Verification items for the finished model (mm, model axes). Give positions to 0.01 mm unless a question says otherwise; leave off trailing zeros. Loops run counter-clockwise (first coordinate to the right, second up) from the corner with the lowest first, then second, coordinate; pieces in that order, holes last. Notation, with made-up numbers: (-24, 49.5) - (10, 49.5) arc R12 cw to (10, 59.5) - close; hole circle Ø8 at (-1.75, 65.5). An arc over 180 degrees is marked (long way). Put each result on its own line as item: value. Start each with the question number.
```python
from build123d import *

# Parameters (mm, degrees)
CHAMFER1_SIZE = 0.5
CHAMFER2_SIZE = 0.5


with BuildPart() as part:
    # Sketch1 → Revolve1 (revolve)
    with BuildSketch(Plane.XY, mode=Mode.PRIVATE) as revolve1_sk:
        with BuildLine():
            Line((5.5, 14.5), (2.236067977, 14.5))
            ThreePointArc((2.236067977, 14.5), (0, 15.5), (-2.236067977, 14.5))
            Line((-2.236067977, 14.5), (-5.5, 14.5))
            Line((-5.5, 14.5), (-5.5, 17.5))
            Line((-5.5, 17.5), (5.5, 17.5))
            Line((5.5, 17.5), (5.5, 14.5))
        make_face()
    revolve(revolve1_sk.sketch.rotate(Axis((-7.5, 0, 0), (1, 0, 0)), 90), axis=Axis((-7.5, 0, 0), (1, 0, 0)))

    # Chamfer1
    chamfer1_edges = [part.edges().sort_by_distance(p)[0] for p in [
        (5.5, 0, -17.5),
        (-5.5, 0, -17.5),
    ]]
    chamfer(chamfer1_edges, length=CHAMFER1_SIZE)

    # Chamfer2
    chamfer2_edges = [part.edges().sort_by_distance(p)[0] for p in [
        (-5.5, 0, -14.5),
        (5.5, 0, -14.5),
    ]]
    chamfer(chamfer2_edges, length=CHAMFER2_SIZE)


solid = part.part
```
1) Section check C-C, the plane x = -2.75. Enter the section's corners in (y, z).
2) Draft check along Y on faces 1 (the face through (0.07, 17.084, -3.794)), 2 (the face through (3.599, 12.864, 6.691)), 3 (the face through (-5.5, 14, -6)). Enter one of: pulls with the +Y half, pulls with the -Y half, needs draft (parallel to the pull), parting line crosses it, or undercut.
3) Scan lines: line 1 along Y through (x, z) = (3.95, 0); line 2 along Y through (x, z) = (3.75, -1.5); line 3 along Z through (x, y) = (2, -6.5). Record each from-to range of solid material in increasing order. Write a range as from..to.
4) Section check A-A, the plane z = 0. Enter the section's corners in (x, y).
5) Depth check by flat-ended pin: P1, Ø5, axis at y = 6.5, z = 10, coming from the -X side; P2, Ø2, axis at x = 4, y = 4.5, coming from the -Z side; P3, Ø3, axis at x = -0.5, z = -1, coming from the +Y side; P4, Ø1.5, axis at x = -1, y = 12, coming from the +Z side. Enter the tip coordinate at first touch or a pass-through.
Results are:
1. outline: circle Ø35 at (0, 0); hole circle Ø29 at (0, 0)
2. face 1: parting line crosses it
2. face 2: undercut
2. face 3: needs draft
3. line 1: y = -17.5..-14.5, 14.5..17.5
3. line 2: y = -17.44..-14.42, 14.42..17.44
3. line 3: z = -16.25..-13.23, 13.23..16.25
4. outline: (-5.5, -17) - (-5, -17.5) - (5, -17.5) - (5.5, -17) - (5.5, -15) - (5, -14.5) - (2.24, -14.5) arc R3 cw to (-2.24, -14.5) - (-5, -14.5) - (-5.5, -15) - close; (-5.5, 15) - (-5, 14.5) - (-2.24, 14.5) arc R3 cw to (2.24, 14.5) - (5, 14.5) - (5.5, 15) - (5.5, 17) - (5, 17.5) - (-5, 17.5) - (-5.5, 17) - close
5. P1: passes through
5. P2: stops at z = -17.15
5. P3: stops at y = 17.5
5. P4: stops at z = 13.4
